Source: CAD feature listing. Evaluate the final solid. Frame: model axes, mm. A direction names the side the tool comes from. Give positions to 0.01 mm unless a question says otherwise; leave off trailing zeros. Order: outer loops, then holes, each group sorted by start corner. A loop starts at its lowest first (then second) coordinate and runs counter-clockwise, first axis right, second up. Notation, with made-up numbers: M 89,20.25 L 136,20.25 A25 ccw 136,32.25 Z; hole C 1.25,53.25 d10. An arc over 180 degrees is marked long. Return JSON: item names as keys, results as strings.
Autodesk Inventor part; units mm, degrees
ref_plane "Start Plane" through (0, 0, -12.7) normal (0, 0, 1) x (1, 0, 0)
ref_plane "End Plane" through (0, 0, 793.75) normal (0, 0, 1) x (1, 0, 0)
ref_plane "Work Plane5" through (-762, -1149.35, 793.75) normal (0, 0, 1) x (1, 0, 0)
ref_plane "Start Plane" through (0, 0, -12.7) normal (0, 0, 1) x (1, 0, 0)
ref_plane "End Plane" through (0, 0, 793.75) normal (0, 0, 1) x (1, 0, 0)
sketch "Sketch" plane through (0, 0, 0) normal (0, 0, 1) x (1, 0, 0)
  line L0 (-19.05, 19.05) -> (19.05, 19.05)
  line L1 (19.05, 19.05) -> (19.05, -19.05)
  line L2 (19.05, -19.05) -> (-19.05, -19.05)
  line L3 (-19.05, -19.05) -> (-19.05, 19.05)
  line L4 (15.875, 15.875) -> (-15.875, 15.875)
  line L5 (-15.875, 15.875) -> (-15.875, -15.875)
  line L6 (-15.875, -15.875) -> (15.875, -15.875)
  line L7 (15.875, -15.875) -> (15.875, 15.875)
  point P0 (0, 0)
  point P1 (0, 19.05)
  point P2 (-19.05, 0)
  dimension "width" = 38.1
  dimension "d1" = 3.175
extrude "Body" add sketch "Sketch" along normal up to surface (806.45 mm away) from surface at -12.7
sketch "Sketch4" plane through (0, 0, 0) normal (0, 0, 1) x (1, 0, 0)
  line L0 (0, 0) -> (10, 0)
ref_plane "Work Plane4" through (0, 0, 0) normal (0, -1, 0) x (1, 0, 0)
sketch "Sketch5" plane through (0, 0, 0) normal (0, -1, 0) x (1, 0, 0)
  line L0 (-2, -12.7) -> (12, -12.7)
  line L1 (-2, 793.75) -> (12, 793.75)
  dimension "d9" = 806.45
ref_plane "Work Plane5" through (-762, -1149.35, 793.75) normal (0, 0, 1) x (1, 0, 0)
split "Split1" plane through (-762, -1149.35, 793.75) removes the side toward (0, 0, 1)
ref_plane "Work Plane6" through (0, 19.05, -12.7) normal (0, 0, -1) x (-1, 0, 0)
split "Split2" plane through (0, 19.05, -12.7) removes the side toward (0, 0, -1)
equation "\"G_OFFSET_START\" = 12.7"
equation "\"G_OFFSET_END\" = -19.05"
equation "\"d4\" = -G_OFFSET_START"
equation "\"d5\" = length + G_OFFSET_END"
equation "\"G_L\" = 812.8"
properties part number "1.5x1.5x.125 Tube" material "Aluminum-6061"
1. Ray query, probe 1 along X at (y, z) = (10.5, 290) (3 decimals). Return the intervals inside material, ascending.
Evaluation:
{"probe 1": "x = -19.05 to -15.875, 15.875 to 19.05"}
2. Set-up query: faces 1 (the face through (15.875, 0, 385)), 2 (the face through (-17, 0, 793.75)). Return all of +Z, -Z, +X, -X, +Y, -Y with unobstructed straight access to the full face (end or side cutting, diameter ignored); none if empty.
Evaluation:
{"face 1": "+Z, -Z", "face 2": "+Z, +X, -X, +Y, -Y"}
3. Section query A-A (y = -7.5). Return loops of the section in (x, z) (3 decimals).
Evaluation:
{"outline": "M -19.05,-12.7 L -15.875,-12.7 L -15.875,793.75 L -19.05,793.75 Z; M 15.875,-12.7 L 19.05,-12.7 L 19.05,793.75 L 15.875,793.75 Z"}
4. Draft query along Y for faces 3 (the face through (0, -15.875, 385)), 4 (the face through (0, 15.875, 385)), 5 (the face through (0, 19.05, 385)), 6 (the face through (-17, 0, -12.7)). Return one class per face: pulls with the +Y half, pulls with the -Y half, needs draft (parallel to the pull), parting line crosses it, or undercut.
Evaluation:
{"face 3": "undercut", "face 4": "undercut", "face 5": "pulls with the +Y half", "face 6": "needs draft"}
5. Section query B-B (z = 389.5). Return loops of the section in (x, y) (3 decimals), then the cut area to 3 significant figures.
Evaluation:
{"outline": "M -19.05,-19.05 L 19.05,-19.05 L 19.05,19.05 L -19.05,19.05 Z; hole M -15.875,-15.875 L 15.875,-15.875 L 15.875,15.875 L -15.875,15.875 Z", "area": "444 mm^2"}
